Check sheet for the modelled part. Datum: model origin and axes. Units: mm. Face numbers are marked on the shaded views. A direction names the side the tool comes from. Give positions to 0.01 mm unless a question says otherwise; leave off trailing zeros. Write each loop counter-clockwise with the first axis right and the second up, starting at its lowest first coordinate (ties: lowest second). Pieces come first, ordered by that corner, then holes.
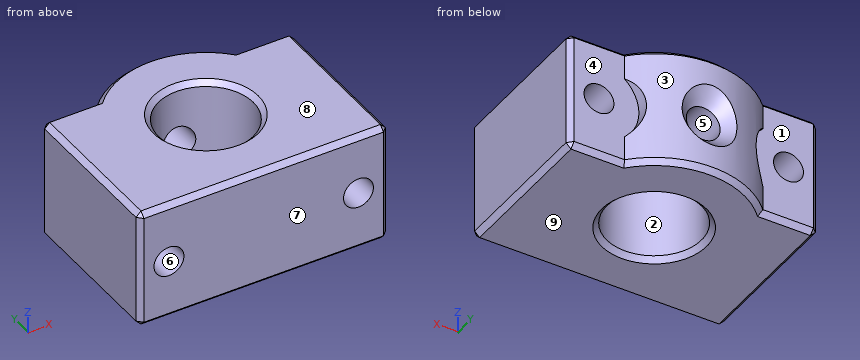
from build123d import *

# Parameters (mm, degrees)
SKETCH1_R                                       = 4.75
BOSS_EXTRUDE1_DEPTH                             = 6
CUT_EXTRUDE1_REACH                              = 23.172
SKETCH2_R                                       = 1.5
CUT_EXTRUDE2_DEPTH                              = 3
CSK_FOR_M3_FLAT_HEAD_MACHINE_SCREW1_D           = 3.4
CSK_FOR_M3_FLAT_HEAD_MACHINE_SCREW1_DEPTH       = 9
CSK_FOR_M3_FLAT_HEAD_MACHINE_SCREW1_CSINK_D     = 6.3
CSK_FOR_M3_FLAT_HEAD_MACHINE_SCREW1_CSINK_ANGLE = 90
CSK_FOR_M3_FLAT_HEAD_MACHINE_SCREW1_TIP         = 1.021463052
CHAMFER1_SIZE                                   = 0.5


with BuildPart() as part:
    # Sketch1 → Boss-Extrude1 (new, symmetric)
    with BuildSketch(Plane.XY):
        with BuildLine():
            Line((6.92820323, 16), (12.5, 16))
            Line((12.5, 16), (12.5, 0))
            Line((12.5, 0), (-12.5, 0))
            Line((-12.5, 0), (-12.5, 16))
            Line((-12.5, 16), (-6.92820323, 16))
            ThreePointArc((-6.92820323, 16), (0, 19), (6.92820323, 16))
        make_face()
        with Locations((0, 9.5)):
            Circle(SKETCH1_R, mode=Mode.SUBTRACT)
    extrude(amount=BOSS_EXTRUDE1_DEPTH, both=True)

    # Sketch2 → Cut-Extrude1 (cut, up to next)
    with BuildSketch(Plane(origin=(0, 16, 0), x_dir=(1, 0, 0), z_dir=(0, 1, 0)), mode=Mode.PRIVATE) as cut_extrude1_sk1:
        with Locations(Location((-9.5, 0, 0), (0, 0, 270))):
            Circle(SKETCH2_R)
    cut_extrude1_tool1 = extrude(cut_extrude1_sk1.sketch, amount=-CUT_EXTRUDE1_REACH, mode=Mode.PRIVATE) & part.part
    # Sketch2 → Cut-Extrude1 (cut, up to next)
    with BuildSketch(Plane(origin=(0, 16, 0), x_dir=(1, 0, 0), z_dir=(0, 1, 0)), mode=Mode.PRIVATE) as cut_extrude1_sk2:
        with Locations(Location((9.5, 0, 0), (0, 0, 270))):
            Circle(SKETCH2_R)
    cut_extrude1_tool2 = extrude(cut_extrude1_sk2.sketch, amount=-CUT_EXTRUDE1_REACH, mode=Mode.PRIVATE) & part.part
    add(cut_extrude1_tool1.solids().sort_by_distance((-9.5, 16, 0))[0], mode=Mode.SUBTRACT)
    add(cut_extrude1_tool2.solids().sort_by_distance((9.5, 16, 0))[0], mode=Mode.SUBTRACT)

    # Sketch3 → Cut-Extrude2 (cut)
    with BuildSketch(Plane(origin=(0, 16, 0), x_dir=(1, 0, 0), z_dir=(0, 1, 0))):
        with BuildLine():
            Line((6.92820323, -3.06363532), (6.92820323, 3.06363532))
            ThreePointArc((6.92820323, 3.06363532), (5.5, 0), (6.92820323, -3.06363532))
        make_face()
        with BuildLine():
            Line((-6.92820323, -3.06363532), (-6.92820323, 3.06363532))
            ThreePointArc((-6.92820323, 3.06363532), (-5.5, 0), (-6.92820323, -3.06363532))
        make_face()
    extrude(amount=CUT_EXTRUDE2_DEPTH, mode=Mode.SUBTRACT)

    # CSK for M3 Flat Head Machine Screw1
    with Locations(Plane(origin=(0, 19, 0), x_dir=(1, 0, 0), z_dir=(0, 1, 0))):
        with Locations((0, 0)):
            CounterSinkHole(CSK_FOR_M3_FLAT_HEAD_MACHINE_SCREW1_D / 2, CSK_FOR_M3_FLAT_HEAD_MACHINE_SCREW1_CSINK_D / 2, depth=CSK_FOR_M3_FLAT_HEAD_MACHINE_SCREW1_DEPTH, counter_sink_angle=CSK_FOR_M3_FLAT_HEAD_MACHINE_SCREW1_CSINK_ANGLE)
            with Locations((0, 0, -(CSK_FOR_M3_FLAT_HEAD_MACHINE_SCREW1_DEPTH + CSK_FOR_M3_FLAT_HEAD_MACHINE_SCREW1_TIP / 2))):  # 118° drill point
                Cone(0, CSK_FOR_M3_FLAT_HEAD_MACHINE_SCREW1_D / 2, CSK_FOR_M3_FLAT_HEAD_MACHINE_SCREW1_TIP, mode=Mode.SUBTRACT)

    # Chamfer1
    chamfer1_edges = [part.edges().sort_by_distance(p)[0] for p in [
        (12.5, 0, 0),
        (-12.5, 0, 0),
        (-12.5, 16, 0),
        (12.5, 16, 0),
        (0, 19, 6),
        (-9.714101615, 16, 6),
        (-4.75, 9.5, -6),
        (-4.75, 9.5, 6),
        (-12.5, 8, 6),
        (0, 0, 6),
        (12.5, 8, 6),
        (0, 0, -6),
        (-12.5, 8, -6),
        (-9.714101615, 16, -6),
        (0, 19, -6),
        (9.714101615, 16, -6),
        (12.5, 8, -6),
        (9.714101615, 16, 6),
    ]]
    chamfer(chamfer1_edges, length=CHAMFER1_SIZE)


solid = part.part
1) Sectioned sample at D-D on x = 0. Record the boundary of the cut face in (y, z).
2) Gauge pin test, flat ends, axial feed: pin 1 (2 mm diameter, centred on x = 0, y = 11.5, fed in from -Z); pin 2 (6 mm diameter, centred on x = -10, z = 0.5, fed in from +Y). Record the tip position at first contact, or that the pin passes through.
3) Draft check along Z on the marked faces 6, 7, 8 and 9. Enter one of: +Z half, -Z half, draft (parallel to the pull), parting line (faces both ways), or undercut.
4) Sectioned sample at B-B on x = -9.5. Record the boundary of the cut face in (y, z), then the cut area to 4 significant figures.
5) Scan lines: L1, parallel to Z at x = 0, y = 14.9; L2, parallel to X at y = 10.5, z = -0.75; L3, parallel to X at y = 10.25, z = 0.25. Record each from-to range of solid material in increasing order.
6) Access from +Z, -Z, +X, -X, +Y, -Y to the whole of each face (thin tool, end or side, straight path). Record for the marked faces 1, 2, 3, 4 and 5.
7) Sectioned sample at C-C on z = -4. Record the boundary of the cut face in (x, y).
8) Sectioned sample at A-A on y = 2. Record the boundary of the cut face in (x, z).
Answers below:
1. outline: (0, -5.5) - (0.5, -6) - (4.25, -6) - (4.75, -5.5) - (4.75, 5.5) - (4.25, 6) - (0.5, 6) - (0, 5.5) - close; (14.25, -5.5) - (14.75, -6) - (18.5, -6) - (19, -5.5) - (19, -3.15) - (17.55, -1.7) - (14.25, -1.7) - close; (14.25, 1.7) - (17.55, 1.7) - (19, 3.15) - (19, 5.5) - (18.5, 6) - (14.75, 6) - (14.25, 5.5) - close
2. pin 1: passes through
2. pin 2: stops at y = 16
3. face 6: undercut
3. face 7: draft
3. face 8: +Z half
3. face 9: -Z half
4. outline: (0, -5.5) - (0.5, -6) - (15.5, -6) - (16, -5.5) - (16, -1.5) - (0, -1.5) - close; (0, 1.5) - (16, 1.5) - (16, 5.5) - (15.5, 6) - (0.5, 6) - (0, 5.5) - close
4. area: 143.5 mm2
5. L1: z = -6 to -1.7, 1.7 to 6
5. L2: x = -12.5 to -10.8, -8.2 to -4.64, 4.64 to 8.2, 10.8 to 12.5
5. L3: x = -12.5 to -10.98, -8.02 to -4.69, 4.69 to 8.02, 10.98 to 12.5
6. face 1: -X, +Y
6. face 2: +Z, -Z
6. face 3: +Z, -Z, +Y
6. face 4: +X, +Y
6. face 5: +Y
7. outline: (-12.5, 0.5) - (-12, 0) - (12, 0) - (12.5, 0.5) - (12.5, 15.5) - (12, 16) - (6.93, 16) arc R9.5 ccw to (-6.93, 16) - (-12, 16) - (-12.5, 15.5) - close; hole circle Ø9.5 at (0, 9.5)
8. outline: (-12.5, -5.5) - (-12, -6) - (12, -6) - (12.5, -5.5) - (12.5, 5.5) - (12, 6) - (-12, 6) - (-12.5, 5.5) - close; hole circle Ø3 at (-9.5, 0); hole circle Ø3 at (9.5, 0)
